Here's how the part is built. I have some questions about the finished solid (model axes, mm). A direction names the side the tool comes from. Round coordinates to 2 decimals unless told otherwise and drop trailing zeros. Write each loop counter-clockwise with the first axis right and the second up, starting at its lowest first coordinate (ties: lowest second). Pieces come first, ordered by that corner, then holes. Notation, with made-up numbers: (-26.75, 60) -> (30.25, 60) arc R9 cw to (30.25, 64) -> close; hole circle Ø5 at (79.25, 63). An arc over 180 degrees is marked (long way). Put each result on its own line as item: value. Start each with the question number.
1. We'd pull the mould along Y, two halves only. Please class faces 6 (the face through (-30.532, -109, 1)), 7 (the face through (-94.68, -122.59, 0.79)), 8 (the face through (-54, -121.326, 3)): +Y half, -Y half, draft (parallel to the pull), parting line (faces both ways), or undercut.
2. I need wall thicknesses on probe 1 along X at (y, z) = (-121, 0.5); probe 2 along X at (y, z) = (-122, 1.75); probe 3 along Y at (x, z) = (-82.5, 3.25). Which ranges of each line are inside material? Lowest first, please. Write a range as from..to.
3. Suppose I cut it at D-D (y = -122). Please give me the cut outline in (x, z), then the cut area to 3 significant figures.
4. Which directions (+Z, -Z, +X, -X, +Y, -Y) give clear straight access to the entire face, cutting with the end or side of a thin tool? Please do faces 1 (the face through (-39.032, -125, 3)), 2 (the face through (-51.632, -124, 3)), 3 (the face through (-63, -99.493, 4)), 4 (the face through (-83, -121.367, 3)), 5 (the face through (-83, -125, 1.6)).
5. Suppose I cut it at A-A (x = -47.5). Please give me the cut outline in (y, z), then the cut area to 3 significant figures.
6. For pin 1 (12 mm diameter, centred on x = -62.5, y = -108.5, fed in from +Z); pin 2 (0.5 mm diameter, centred on y = -106, z = 0.5, fed in from -X); pin 3 (5 mm diameter, centred on x = -83, y = -124, fed in from +Z), each with a flat end and sliding along its axis, tell me the tip position at first contact or that it passes through.
7. Suppose I cut it at C-C (z = 5.75). Please give me the cut outline in (x, y), then the cut area to 3 significant figures.
8. Suppose I cut it at B-B (y = -112). Please give me the cut outline in (x, z), then the cut area to 3 significant figures.
```python
from build123d import *

# Parameters (mm, degrees)
F0_R     = 1.375
F1_DEPTH = 1.6
F2_W     = 2.44764
F2_H     = 15
F2_W_2   = 3.340326
F3_DEPTH = 2
F2_W_3   = 50
F2_H_2   = 5
F4_DEPTH = 5
F2_W_4   = 5
F2_H_3   = 2.543583
F2_H_4   = 2.167234
F2_H_5   = 2.553497
F2_H_6   = 5.309687
F5_DEPTH = 2
F2_W_5   = 10
F2_H_7   = 2.125936
F6_DEPTH = 3


with BuildPart() as f1:
    # F0 (on Top) → F1 (new body)
    with BuildSketch(Plane.XY):
        with BuildLine():
            Line((-33.531875, -93.493047), (-92.531875, -93.493047))
            ThreePointArc((-92.531875, -93.493047), (-94.653195, -94.371726), (-95.531875, -96.493047))
            Line((-95.531875, -96.493047), (-95.531875, -120.493047))
            ThreePointArc((-95.531875, -120.493047), (-94.653195, -122.614367), (-92.531875, -123.493047))
            Line((-92.531875, -123.493047), (-33.531875, -123.493047))
            ThreePointArc((-33.531875, -123.493047), (-31.410555, -122.614367), (-30.531875, -120.493047))
            Line((-30.531875, -120.493047), (-30.531875, -96.493047))
            ThreePointArc((-30.531875, -96.493047), (-31.410555, -94.371726), (-33.531875, -93.493047))
        make_face()
        with Locations((-92.031875, -119.993047)):
            Circle(F0_R, mode=Mode.SUBTRACT)
        with Locations((-34.031875, -119.993047)):
            Circle(F0_R, mode=Mode.SUBTRACT)
        with Locations((-92.031875, -96.993047)):
            Circle(F0_R, mode=Mode.SUBTRACT)
        with Locations((-34.031875, -96.993047)):
            Circle(F0_R, mode=Mode.SUBTRACT)
    extrude(amount=F1_DEPTH)

    # F2 (on face) → F3 (join)
    with BuildSketch(Plane.XY.offset(1.6)):
        with Locations((-96.755695, -106.593047)):
            Rectangle(F2_W, F2_H)
        with Locations((-93.861712, -106.593047)):
            Rectangle(F2_W_2, F2_H)
    extrude(amount=F3_DEPTH)

    # F2 (on face) → F4 (join)
    with BuildSketch(Plane.XY.offset(1.6)):
        with Locations((-63.031875, -96.993047)):
            Rectangle(F2_W_3, F2_H_2)
    extrude(amount=F4_DEPTH)

    # F2 (on face) → F5 (join)
    with BuildSketch(Plane.XY.offset(1.6)):
        with Locations((-54.131875, -124.764838)):
            Rectangle(F2_W_4, F2_H_3)
        with Locations((-54.131875, -122.40943)):
            Rectangle(F2_W_4, F2_H_4)
        with Locations((-41.531875, -122.216298)):
            Rectangle(F2_W_4, F2_H_5)
        with Locations((-41.531875, -126.14789)):
            Rectangle(F2_W_4, F2_H_6)
    extrude(amount=F5_DEPTH)

    # F2 (on face) → F6 (join)
    with BuildSketch(Plane.XY.offset(1.6)):
        with Locations((-83.131875, -122.430079)):
            Rectangle(F2_W_5, F2_H_7)
        with Locations((-83.131875, -124.764838)):
            Rectangle(F2_W_5, F2_H_3)
    extrude(amount=F6_DEPTH)


solid = f1.part
```
Verdict:
1. face 6: draft
1. face 7: -Y half
1. face 8: undercut
2. probe 1: x = -95.49..-92.97, -91.1..-34.97, -33.1..-30.58
2. probe 2: x = -88.13..-78.13, -56.63..-51.63, -44.03..-39.03
2. probe 3: y = -126.04..-121.37, -99.49..-94.49
3. outline: (-95.13, 0) -> (-30.94, 0) -> (-30.94, 1.6) -> (-39.03, 1.6) -> (-39.03, 3.6) -> (-44.03, 3.6) -> (-44.03, 1.6) -> (-51.63, 1.6) -> (-51.63, 3.6) -> (-56.63, 3.6) -> (-56.63, 1.6) -> (-78.13, 1.6) -> (-78.13, 4.6) -> (-88.13, 4.6) -> (-88.13, 1.6) -> (-95.13, 1.6) -> close
3. area: 153 mm^2
4. face 1: +Z, +X, -Y
4. face 2: +Z, -Y
4. face 3: +Z, +X
4. face 4: +Z, -X
4. face 5: -Z, +X, -X, -Y
5. outline: (-123.49, 0) -> (-93.49, 0) -> (-93.49, 1.6) -> (-94.49, 1.6) -> (-94.49, 6.6) -> (-99.49, 6.6) -> (-99.49, 1.6) -> (-123.49, 1.6) -> close
5. area: 73.0 mm^2
6. pin 1: stops at z = 1.6
6. pin 2: stops at x = -95.53
6. pin 3: stops at z = 4.6
7. outline: (-88.03, -99.49) -> (-38.03, -99.49) -> (-38.03, -94.49) -> (-88.03, -94.49) -> close
7. area: 250 mm^2
8. outline: (-97.98, 1.6) -> (-95.53, 1.6) -> (-95.53, 0) -> (-30.53, 0) -> (-30.53, 1.6) -> (-92.19, 1.6) -> (-92.19, 3.6) -> (-97.98, 3.6) -> close
8. area: 116 mm^2
